Here's how the part is built. I have some questions about the finished solid (model axes, mm). A direction names the side the tool comes from. Coordinates: 2 decimals unless noted, no trailing zeros. Write each loop counter-clockwise with the first axis right and the second up, starting at its lowest first coordinate (ties: lowest second). Pieces come first, ordered by that corner, then holes.
Autodesk Inventor part; units mm, degrees
ref_plane "YZ Plane" through (0, 0, 0) normal (1, 0, 0) x (0, 1, 0)
ref_plane "XZ Plane" through (0, 0, 0) normal (0, 1, 0) x (-1, 0, 0)
ref_plane "XY Plane" through (0, 0, 0) normal (0, 0, 1) x (1, 0, 0)
sketch "Эскиз1" plane through (0, 0, 0) normal (0, 0, 1) x (1, 0, 0)
  line L0 (-5.1487, -13.4444) -> (-9.7487, -13.4444)
  line L1 (-9.7487, -13.4444) -> (-9.7487, -18.4444)
  line L2 (-9.7487, -18.4444) -> (7.2513, -18.4444)
  line L3 (7.2513, -18.4444) -> (7.2513, -13.4444)
  line L4 (7.2513, -13.4444) -> (2.6513, -13.4444)
  line L5 (2.6513, -13.4444) -> (2.6513, -8.4651)
  line L6 (2.6513, -8.4651) -> (7.2513, -8.4651)
  line L7 (7.2513, -8.4651) -> (7.2513, 21.5556)
  line L8 (7.2513, 21.5556) -> (-9.7487, 21.5556)
  line L9 (-9.7487, 21.5556) -> (-9.7487, -8.4237)
  line L10 (-9.7487, -8.4237) -> (-5.1487, -8.4237)
  line L11 (-5.1487, -8.4237) -> (-5.1487, -13.4444)
  circle A0 centre (-1.2487, 17.5556) radius 1
extrude "Выдавливание1" add sketch "Эскиз1" along normal blind 4.9
properties part number "В. шарн. - держатель смартфона"
1. Thinking about a two-plate mould opening in X: for faces 4 (the face through (-9.749, -16, 2)), 5 (the face through (-1.379, 16.564, 2.416)), 6 (the face through (-1, 21.556, 2)), 7 (the face through (2.651, -11, 2)), which applies, pulls with the +X half, pulls with the -X half, needs draft (parallel to the pull), parting line crosses it, or undercut?
2. I want a section at B-B (z = 2.1). List the corners of the cut face in (x, y) for me, then the cut area to 3 significant figures.
3. I want a section at A-A (x = -7.25). List the corners of the cut face in (y, z) for me, then the cut area to 3 significant figures.
4. I want a section at C-C (x = 4.75). List the corners of the cut face in (y, z) for me.
5. On a 3-axis mill with a long thin cutter (end or side, diameter ignored), from which of +Z, -Z, +X, -X, +Y, -Y can I reach the whole of each face in a straight line? I mean faces 1 (the face through (7.251, -16, 2)), 2 (the face through (5, -8.465, 2)), 3 (the face through (-5.149, -11, 2)). Say none if no direction works.
6. I want a section at D-D (y = -13). List the corners of the cut face in (x, z) for me, then the cut area to 3 significant figures.
7. If I drill on line 1 (Y direction, x = -9, z = 3.15); line 2 (Y direction, x = 5.75, z = 2.5); line 3 (X direction, y = 18, z = 3.85), over which ranges is the centre line in solid material (lowest first)?
8. For pin 1 Ø2.5 at (y, z) = (-11, 3.5) entering from +X, with a flat end and sliding along its axis, tell me the tip position at first contact or that it passes through.
Response values:
1. face 4: pulls with the -X half
1. face 5: undercut
1. face 6: needs draft
1. face 7: pulls with the +X half
2. outline: (-9.75, -18.44) - (7.25, -18.44) - (7.25, -13.44) - (2.65, -13.44) - (2.65, -8.47) - (7.25, -8.47) - (7.25, 21.56) - (-9.75, 21.56) - (-9.75, -8.42) - (-5.15, -8.42) - (-5.15, -13.44) - (-9.75, -13.44) - close; hole circle Ø2 at (-1.25, 17.56)
2. area: 631 mm2
3. outline: (-18.44, 0) - (-13.44, 0) - (-13.44, 4.9) - (-18.44, 4.9) - close; (-8.42, 0) - (21.56, 0) - (21.56, 4.9) - (-8.42, 4.9) - close
3. area: 171 mm2
4. outline: (-18.44, 0) - (-13.44, 0) - (-13.44, 4.9) - (-18.44, 4.9) - close; (-8.47, 0) - (21.56, 0) - (21.56, 4.9) - (-8.47, 4.9) - close
5. face 1: +Z, -Z, +X, +Y, -Y
5. face 2: +Z, -Z, +X
5. face 3: +Z, -Z, -X
6. outline: (-5.15, 0) - (2.65, 0) - (2.65, 4.9) - (-5.15, 4.9) - close
6. area: 38.2 mm2
7. line 1: y = -18.44 to -13.44, -8.42 to 21.56
7. line 2: y = -18.44 to -13.44, -8.47 to 21.56
7. line 3: x = -9.75 to -2.14, -0.35 to 7.25
8. pin 1: stops at x = 2.65
